Geometry: see drawing. Coordinates: mm, zero at the bounding-box minimum. A direction names the side the tool comes from. Round coordinates to 2 decimals unless told otherwise and drop trailing zeros. Loops run counter-clockwise (first coordinate to the right, second up) from the corner with the lowest first, then second, coordinate; pieces in that order, holes last. Notation, with made-up numbers: M 58,83 L 82,83 A17 ccw 82,89 Z; hole C 70.5,9.5 d7. An arc over 180 degrees is marked long. Answer as a JSON object with one key per item and string values.
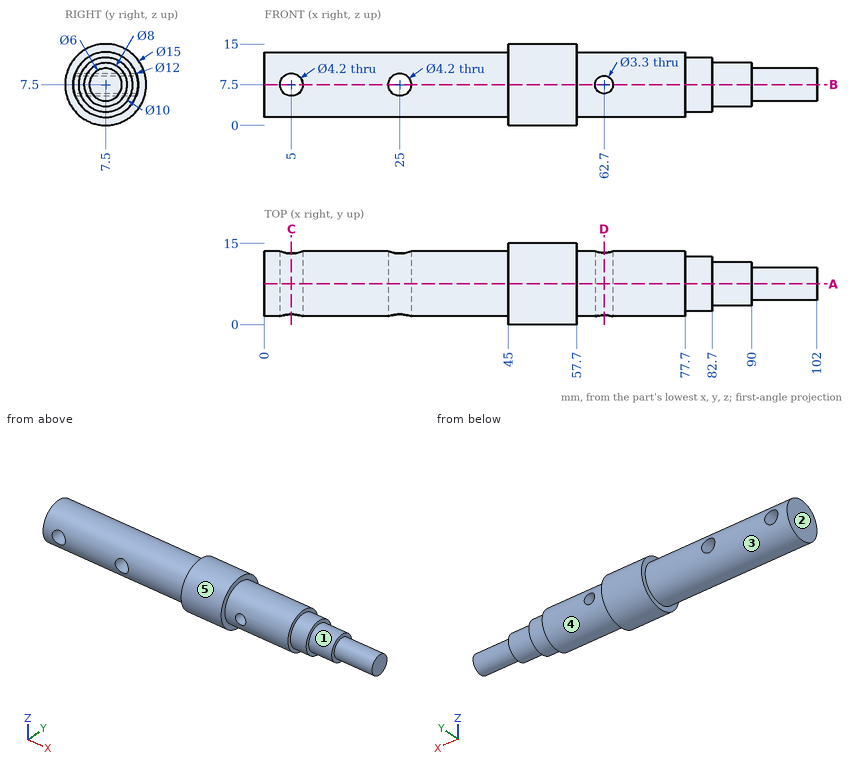
1) Pull-direction query (Y, two-part tool) for the marked faces 1 and 2; classes: +Y half, -Y half, draft (parallel to the pull), parting line (faces both ways), or undercut.
Results:
{"face 1": "parting line", "face 2": "draft"}
2) Pin query (flat end, axial travel): P1, Ø5.5, axis at x = 25, z = 7.5, coming from the -Y side; P2, Ø2, axis at x = 89.5, z = 10.5, coming from the +Y side; P3, Ø4, axis at x = 62.7, z = 7.5, coming from the +Y side. Return the tip coordinate at first contact, or that it passes through.
Results:
{"P1": "y = 1.5", "P2": "y = 10.96", "P3": "y = 13.5"}
3) Section query A-A (y = 7.5). Return the cut outline in (x, z).
Results:
{"outline": "M 0,1.5 L 45,1.5 L 45,0 L 57.7,0 L 57.7,1.5 L 77.7,1.5 L 77.7,2.5 L 82.7,2.5 L 82.7,3.5 L 90,3.5 L 90,4.5 L 102,4.5 L 102,10.5 L 90,10.5 L 90,11.5 L 82.7,11.5 L 82.7,12.5 L 77.7,12.5 L 77.7,13.5 L 57.7,13.5 L 57.7,15 L 45,15 L 45,13.5 L 0,13.5 Z; hole C 5,7.5 d4.2; hole C 25,7.5 d4.2; hole C 62.7,7.5 d3.3"}
4) Reachability of the marked faces 3, 4 and 5 from +Z, -Z, +X, -X, +Y, -Y: full face, straight path, thin tool, end or side. Return the list, or none.
Results:
{"face 3": "-X", "face 4": "+X", "face 5": "+X, -X"}
5) Section query C-C (x = 5). Return the cut outline in (y, z), and give its area (3 significant figures).
Results:
{"outline": "M 1.88,5.4 A6 ccw 13.12,5.4 Z; M 1.88,9.6 L 13.12,9.6 A6 ccw Z", "area": "63.7 mm2"}
6) Section query D-D (x = 62.7). Return the cut outline in (y, z).
Results:
{"outline": "M 1.73,5.85 A6 ccw 13.27,5.85 Z; M 1.73,9.15 L 13.27,9.15 A6 ccw Z"}
7) Ray query, line 1 (X direction, y = 6.5, z = 7.5); line 2 (X direction, y = 6, z = 9.25); line 3 (X direction, y = 11.25, z = 8.75). Return the intervals inside material, ascending.
Results:
{"line 1": "0 to 2.9, 7.1 to 22.9, 27.1 to 61.05, 64.35 to 102", "line 2": "0 to 3.84, 6.16 to 23.84, 26.16 to 102", "line 3": "0 to 3.31, 6.69 to 23.31, 26.69 to 61.62, 63.78 to 90"}
8) Section query B-B (z = 7.5). Count the separate pieces of the cut face and the enclosed holes in it, and give its area (3 significant figures).
Results:
{"separate pieces": "4", "enclosed holes": "0", "area": "1,010 mm2"}
